```python
from build123d import *

# Parameters (mm, degrees)
SKETCH_1_W      = 50
SKETCH_1_H      = 12
SKETCH_1_W_2    = 6
SKETCH_1_H_2    = 20
EXTRUDE_1_DEPTH = 6


with BuildPart() as part:
    # 草图1 → 凸台-拉伸1 (new body)
    with BuildSketch(Plane.XY):
        Polygon((-99.950071484, 5.412625096), (-99.950071484, -14.587374904), (-93.950071484, -14.587374904), (-93.950071484, -34.587374904), (-99.950071484, -34.587374904), (-99.950071484, -54.587374904), (-93.950071484, -54.587374904), (-93.950071484, -74.587374904), (-99.950071484, -74.587374904), (-99.950071484, -94.587374904), (-93.950071484, -94.587374904), (-93.950071484, -129.587374904), (194.049928516, -129.587374904), (194.049928516, -94.587374904), (200.049928516, -94.587374904), (200.049928516, -74.587374904), (194.049928516, -74.587374904), (194.049928516, -54.587374904), (200.049928516, -54.587374904), (200.049928516, -34.587374904), (194.049928516, -34.587374904), (194.049928516, -14.587374904), (200.049928516, -14.587374904), (200.049928516, 5.412625096), (194.049928516, 5.412625096), (194.049928516, 25.412625096), (200.049928516, 25.412625096), (200.049928516, 45.412625096), (194.049928516, 45.412625096), (194.049928516, 65.412625096), (200.049928516, 65.412625096), (200.049928516, 85.412625096), (194.049928516, 85.412625096), (194.049928516, 105.412625096), (200.049928516, 105.412625096), (200.049928516, 120.412625096), (194.049928516, 120.412625096), (-93.950071484, 120.412625096), (-99.950071484, 120.412625096), (-99.950071484, 105.412625096), (-93.950071484, 105.412625096), (-93.950071484, 85.412625096), (-99.950071484, 85.412625096), (-99.950071484, 65.412625096), (-93.950071484, 65.412625096), (-93.950071484, 45.412625096), (-99.950071484, 45.412625096), (-99.950071484, 25.412625096), (-93.950071484, 25.412625096), (-93.950071484, 5.412625096), align=None)
        with Locations((100.049928516, -103.587374904)):
            Rectangle(SKETCH_1_W, SKETCH_1_H, mode=Mode.SUBTRACT)
        with Locations((153.049928516, 15.412625096)):
            Rectangle(SKETCH_1_W_2, SKETCH_1_H_2, mode=Mode.SUBTRACT)
        with Locations((153.049928516, -64.587374904)):
            Rectangle(SKETCH_1_W_2, SKETCH_1_H_2, mode=Mode.SUBTRACT)
        with Locations((153.049928516, 55.412625096)):
            Rectangle(SKETCH_1_W_2, SKETCH_1_H_2, mode=Mode.SUBTRACT)
        with Locations((153.049928516, -104.587374904)):
            Rectangle(SKETCH_1_W_2, SKETCH_1_H_2, mode=Mode.SUBTRACT)
        with Locations((153.049928516, 95.412625096)):
            Rectangle(SKETCH_1_W_2, SKETCH_1_H_2, mode=Mode.SUBTRACT)
        with Locations((153.049928516, -24.587374904)):
            Rectangle(SKETCH_1_W_2, SKETCH_1_H_2, mode=Mode.SUBTRACT)
        with Locations((-52.950071484, -24.587374904)):
            Rectangle(SKETCH_1_W_2, SKETCH_1_H_2, mode=Mode.SUBTRACT)
        with Locations((-52.950071484, -64.587374904)):
            Rectangle(SKETCH_1_W_2, SKETCH_1_H_2, mode=Mode.SUBTRACT)
        with Locations((-52.950071484, -104.587374904)):
            Rectangle(SKETCH_1_W_2, SKETCH_1_H_2, mode=Mode.SUBTRACT)
        with Locations((-52.950071484, 55.412625096)):
            Rectangle(SKETCH_1_W_2, SKETCH_1_H_2, mode=Mode.SUBTRACT)
        with Locations((-52.950071484, 95.412625096)):
            Rectangle(SKETCH_1_W_2, SKETCH_1_H_2, mode=Mode.SUBTRACT)
        with Locations((-52.950071484, 15.412625096)):
            Rectangle(SKETCH_1_W_2, SKETCH_1_H_2, mode=Mode.SUBTRACT)
        with Locations((0.049928516, -103.587374904)):
            Rectangle(SKETCH_1_W, SKETCH_1_H, mode=Mode.SUBTRACT)
    extrude(amount=EXTRUDE_1_DEPTH)


solid = part.part
```
For this review, take the finished solid that the model builds, in its own axes (mm). A direction names the side the tool comes from. Give positions to 0.01 mm unless a question says otherwise; leave off trailing zeros. Loops run counter-clockwise (first coordinate to the right, second up) from the corner with the lowest first, then second, coordinate; pieces in that order, holes last. Notation, with made-up numbers: M 69,45 L 86,45 A15 ccw 86,62 Z; hole C 52.25,5.25 d3. An arc over 180 degrees is marked long. One line per item, written item: value. Start each with the question number.
Q1. Draft analysis for pull direction Y (two halves, no side actions). For faces 1 (the face through (48, -129.587, 3)), 2 (the face through (0, -97.587, 3)), 3 (the face through (200.05, 113, 3)), state which applies: released by +Y, released by -Y, zero draft, split by the parting line, or undercut.
Q2. Add section A-A (y = -69). Give the boundary of the cut face in (x, z), and give its area (3 significant figures).
Q3. For L1, parallel to X at y = 10, z = 5.3; L2, parallel to Y at x = 78, z = 3.6, list the stretches that pass through material, from the lowest coordinate up.
Q4. Add section B-B (x = 119). Give the boundary of the cut face in (y, z).
Q5. Machinability: for faces 4 (the face through (-97, -94.587, 3)), 5 (the face through (197, 85.413, 3)), 6 (the face through (153, -54.587, 3)), which of the approach directions +Z, -Z, +X, -X, +Y, -Y give a long, thin tool a straight path to every point of the face, cutting with its end or side? Answer none if there is none.
Q6. Clearance check with flat-ended pins moving along their axes: pin 1 Ø3 at (y, z) = (-29, 4) entering from +X; pin 2 Ø3 at (y, z) = (-68, 3) entering from -X; pin 3 Ø1.8 at (x, z) = (-97, 3.5) entering from -Y. State where each tip first meets the part, or that it passes through.
Q7. Add section C-C (z = 2.9). Count the separate pieces of the cut face and the enclosed holes in it, and give its area (3 significant figures).
Reply:
1. face 1: released by -Y
1. face 2: undercut
1. face 3: zero draft
2. outline: M -93.95,0 L -55.95,0 L -55.95,6 L -93.95,6 Z; M -49.95,0 L 150.05,0 L 150.05,6 L -49.95,6 Z; M 156.05,0 L 194.05,0 L 194.05,6 L 156.05,6 Z
2. area: 1,660 mm²
3. L1: -93.95 to -55.95, -49.95 to 150.05, 156.05 to 194.05
3. L2: -129.59 to -109.59, -97.59 to 120.41
4. outline: M -129.59,0 L -109.59,0 L -109.59,6 L -129.59,6 Z; M -97.59,0 L 120.41,0 L 120.41,6 L -97.59,6 Z
5. face 4: +Z, -Z, -X, -Y
5. face 5: +Z, -Z, +X
5. face 6: +Z, -Z
6. pin 1: x = 194.05
6. pin 2: x = -93.95
6. pin 3: y = -94.59
7. separate pieces: 1
7. enclosed holes: 14
7. area: 70,700 mm²
